Can you work these out from the model? Positions are in its coordinate system, mm. Face numbers are marked on the shaded views. A direction names the side the tool comes from. Give positions to 0.01 mm unless a question says otherwise; leave off trailing zeros. Order: outer loops, then holes, each group sorted by start corner. A loop starts at its lowest first (then second) coordinate and runs counter-clockwise, first axis right, second up.
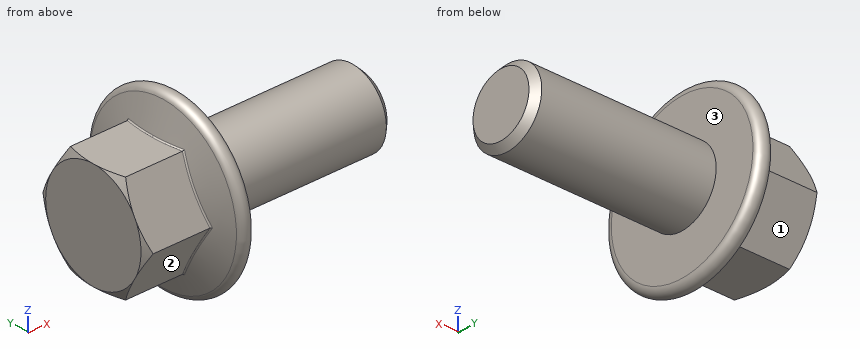
```python
from build123d import *

# Parameters (mm, degrees)
BASEHEAD_DEPTH    = 5.6
FLANGEHEXFILLET_R = 0.1


with BuildPart() as part:
    # Sketch1 → BaseHead (new body)
    with BuildSketch(Plane(origin=(0, 0, 0), x_dir=(0, 0, -1), z_dir=(1, 0, 0))):
        Polygon((3.5, 2.020725942), (3.5, -2.020725942), (0, -4.041451884), (-3.5, -2.020725942), (-3.5, 2.020725942), (0, 4.041451884), align=None)
    extrude(amount=BASEHEAD_DEPTH)

    # BodySke → BaseBody (revolve)
    with BuildSketch(Plane.XY, mode=Mode.PRIVATE) as basebody_sk:
        Polygon((0, 0), (17.6, 0), (17.6, 2.055), (17.155, 2.5), (0, 2.5), align=None)
    revolve(basebody_sk.sketch.rotate(Axis((0, 0, 0), (1, 0, 0)), 90), axis=Axis((0, 0, 0), (1, 0, 0)))

    # Sketch3 → HeadChamfer (revolve, cut)
    with BuildSketch(Plane.XY, mode=Mode.PRIVATE) as headchamfer_sk:
        Polygon((0, 3.5), (3.199358737, 9.041451884), (3.199358737, 14.041451884), (-10, 14.041451884), (-10, 3.5), align=None)
    revolve(headchamfer_sk.sketch.rotate(Axis((0, 0, 0), (1, 0, 0)), 90), axis=Axis((0, 0, 0), (1, 0, 0)), mode=Mode.SUBTRACT)

    # Sketch4 → Flange (revolve)
    with BuildSketch(Plane.XY, mode=Mode.PRIVATE) as flange_sk:
        with BuildLine():
            Line((2.675265896, 0), (4.63015369, 5.371010072))
            ThreePointArc((4.63015369, 5.371010072), (5.186824089, 5.692403877), (5.6, 5.2))
            Line((5.6, 5.2), (5.6, 0))
            Line((5.6, 0), (2.675265896, 0))
        make_face()
    revolve(flange_sk.sketch.rotate(Axis((0, 0, 0), (1, 0, 0)), 90), axis=Axis((0, 0, 0), (1, 0, 0)))

    # FlangeHexFillet
    flangehexfillet_edges = [part.edges().sort_by_distance(p)[0] for p in [
        (3.949161716, 0, -3.5),
        (3.949161716, -3.031088913, -1.75),
        (4.001624527, 1.014770503, 3.5),
        (3.949161716, 3.031088913, 1.75),
        (3.949161716, 3.031088913, -1.75),
        (3.949161716, -3.031088913, 1.75),
        (4.001624527, -1.014770503, 3.5),
    ]]
    fillet(flangehexfillet_edges, radius=FLANGEHEXFILLET_R)


solid = part.part
```
1) Suppose I cut it at B-B (x = 2). Please give me the cut outline in (y, z).
2) Which directions (+Z, -Z, +X, -X, +Y, -Y) give clear straight access to the entire face, cutting with the end or side of a thin tool? Please do the marked faces 1, 2 and 3.
3) If I drill on line 1 (X direction, y = -2, z = 4.25); line 2 (X direction, y = 1, z = 2); line 3 (Y direction, x = 13, z = -0.75), over which ranges is the centre line in solid material (lowest first)?
4) I'm going to push flat-ended pins straight in: pin 1 Ø1.5 at (x, z) = (5.5, 1) entering from -Y; pin 2 Ø5 at (x, z) = (9.5, 1.5) entering from +Y; pin 3 Ø1.5 at (x, z) = (9, 3) entering from -Y. Where does each tip first touch, or does it pass through?
5) Suppose I cut it at A-A (x = 11.25). Please give me the cut outline in (y, z).
Results:
1. outline: (-4.04, 0) - (-2.02, -3.5) - (2.02, -3.5) - (4.04, 0) - (2.02, 3.5) - (-2.02, 3.5) - close
2. face 1: -Z, -X, +Y
2. face 2: -Z, -X, -Y
2. face 3: +X
3. line 1: x = 4.38 to 5.6
3. line 2: x = 0 to 17.42
3. line 3: y = -2.38 to 2.38
4. pin 1: stops at y = -5.69
4. pin 2: stops at y = 2.5
4. pin 3: stops at y = -1.09
5. outline: circle Ø5 at (0, 0)
